```python
from build123d import *

# Parameters (mm, degrees)
BOSS_EXTRUDE1_DEPTH  = 12.7
MIRROR2_COPY_1_DEPTH = 12.7
SKETCH2_R            = 5.08
CUT_EXTRUDE1_DEPTH   = 6.35


with BuildPart() as part:
    # Sketch1 → Boss-Extrude1 (new body)
    with BuildSketch(Plane.XY):
        Polygon((0, 0), (-15.3924, 0), (-10.3124, 8.89), (-8.89, 8.89), (-8.89, 25.908), (0, 30.988), align=None)
    boss_extrude1 = extrude(amount=BOSS_EXTRUDE1_DEPTH)

    # Mirror1: Boss-Extrude1 across plane
    add(boss_extrude1.mirror(Plane(origin=(0, 30.988, 12.7), x_dir=(0, 0, 1), z_dir=(-1, 0, 0))))

    # Mirror2: Boss-Extrude1 across plane
    add(boss_extrude1.mirror(Plane(origin=(0, 0, 12.7), x_dir=(0, 0, 1), z_dir=(0, 1, 0))))

    # Mirror2 copy 1 sketch → Mirror2 copy 1 (add)
    with BuildSketch(Plane(origin=(0, 0, 0), x_dir=(-1, 0, 0), z_dir=(0, 0, 1))):
        Polygon((0, 0), (-15.3924, 0), (-10.3124, 8.89), (-8.89, 8.89), (-8.89, 25.908), (0, 30.988), align=None)
    extrude(amount=MIRROR2_COPY_1_DEPTH)

    # Sketch2 → Cut-Extrude1 (cut)
    with BuildSketch(Plane.XY.offset(12.7)):
        Circle(SKETCH2_R)
    extrude(amount=-CUT_EXTRUDE1_DEPTH, mode=Mode.SUBTRACT)


solid = part.part
```
Geometry check sheet. Reference: the model listing, model coordinates, mm. A direction names the side the tool comes from. Round coordinates to 2 decimals unless told otherwise and drop trailing zeros. Write each loop counter-clockwise with the first axis right and the second up, starting at its lowest first coordinate (ties: lowest second). Pieces come first, ordered by that corner, then holes. Notation, with made-up numbers: (19, 85.5) -> (44, 85.5) arc R14 ccw to (44, 96.5) -> close; hole circle Ø7 at (65.5, 40.5). An arc over 180 degrees is marked (long way). Put each result on its own line as item: value.
1) Access from +Z, -Z, +X, -X, +Y, -Y to the whole of each face (thin tool, end or side, straight path). Record for faces 5 (the face through (0, 6, 12.7)), 6 (the face through (-10, 8.89, 6)), 7 (the face through (0, 0, 6.35)), 8 (the face through (8.89, 17, 6)), 9 (the face through (-10, -8.89, 6)).
Recorded:
face 5: +Z, +X, -X, +Y, -Y
face 6: +Z, -Z, -X, +Y
face 7: +Z
face 8: +Z, -Z, +X, +Y
face 9: +Z, -Z, -X, -Y
2) Release check for a two-part mould opening along Y. For faces 1 (the face through (-0.661, 5.037, 9.569)), 2 (the face through (10, -8.89, 6)), 3 (the face through (-4.51, 28.41, 6.26)), 4 (the face through (8.89, -17, 6)) record: pulls with the +Y half, pulls with the -Y half, needs draft (parallel to the pull), parting line crosses it, or undercut.
Recorded:
face 1: undercut
face 2: pulls with the -Y half
face 3: pulls with the +Y half
face 4: needs draft
3) Cross-section at A-A, the plane z = 8.75. Enter the section's corners in (x, y), plus the area to 3 significant figures.
Recorded:
outline: (-15.39, 0) -> (-10.31, -8.89) -> (-8.89, -8.89) -> (-8.89, -25.91) -> (0, -30.99) -> (8.89, -25.91) -> (8.89, -8.89) -> (10.31, -8.89) -> (15.39, 0) -> (10.31, 8.89) -> (8.89, 8.89) -> (8.89, 25.91) -> (0, 30.99) -> (-8.89, 25.91) -> (-8.89, 8.89) -> (-10.31, 8.89) -> close; hole circle Ø10.16 at (0, 0)
area: 1,070 mm2
4) Thickness scan on probe 1 along Y at (x, z) = (0, 10.25); probe 2 along X at (y, z) = (-15.5, 9.25); probe 3 along Y at (x, z) = (0.5, 7). Record the ranges inside material, lowest first. Write a range as from..to.
Recorded:
probe 1: y = -30.99..-5.08, 5.08..30.99
probe 2: x = -8.89..8.89
probe 3: y = -30.7..-5.06, 5.06..30.7
5) Cross-section at B-B, the plane z = 3.75. Enter the section's corners in (x, y), plus the area to 3 significant figures.
Recorded:
outline: (-15.39, 0) -> (-10.31, -8.89) -> (-8.89, -8.89) -> (-8.89, -25.91) -> (0, -30.99) -> (8.89, -25.91) -> (8.89, -8.89) -> (10.31, -8.89) -> (15.39, 0) -> (10.31, 8.89) -> (8.89, 8.89) -> (8.89, 25.91) -> (0, 30.99) -> (-8.89, 25.91) -> (-8.89, 8.89) -> (-10.31, 8.89) -> close
area: 1,150 mm2
6) Cross-section at D-D, the plane x = 2. Enter the section's corners in (y, z).
Recorded:
outline: (-29.85, 0) -> (29.85, 0) -> (29.85, 12.7) -> (4.67, 12.7) -> (4.67, 6.35) -> (-4.67, 6.35) -> (-4.67, 12.7) -> (-29.85, 12.7) -> close
7) Depth check by flat-ended pin: P1, Ø3, axis at x = -2, y = -0.5, coming from the +Z side; P2, Ø6.5, axis at y = 18.5, z = 5, coming from the -X side; P3, Ø0.7, axis at x = -9.5, z = 6, coming from the +Y side. Enter the tip coordinate at first touch or a pass-through.
Recorded:
P1: stops at z = 6.35
P2: stops at x = -8.89
P3: stops at y = 8.89
8) Cross-section at C-C, the plane y = -3. Enter the section's corners in (x, z).
Recorded:
outline: (-13.68, 0) -> (13.68, 0) -> (13.68, 12.7) -> (4.1, 12.7) -> (4.1, 6.35) -> (-4.1, 6.35) -> (-4.1, 12.7) -> (-13.68, 12.7) -> close
